```python
from build123d import *

# Parameters (mm, degrees)
F0_W     = 50
F0_H     = 50
F1_DEPTH = 400
F2_W     = 30
F2_H     = 30
F3_DEPTH = 40
F4_W     = 30
F4_H     = 10
F5_DEPTH = 30


with BuildPart() as f1:
    # F0 (on Top) → F1 (new body)
    with BuildSketch(Plane.XY):
        with Locations((-25, -25)):
            Rectangle(F0_W, F0_H)
    extrude(amount=-F1_DEPTH)

    # F2 (on face) → F3 (join)
    with BuildSketch(Plane.XY):
        with Locations((-25, -25)):
            Rectangle(F2_W, F2_H)
    extrude(amount=F3_DEPTH)

    # F4 (on face) → F5 (cut)
    with BuildSketch(Plane.XY.offset(40)):
        with Locations((-25, -35)):
            Rectangle(F4_W, F4_H)
        with Locations((-25, -15)):
            Rectangle(F4_W, F4_H)
    extrude(amount=-F5_DEPTH, mode=Mode.SUBTRACT)


solid = f1.part
```
Design review of the part built by this model. Coordinates are the model's own, in mm. A direction names the side the tool comes from. Round coordinates to 2 decimals unless told otherwise and drop trailing zeros. Order: outer loops, then holes, each group sorted by start corner. A loop starts at its lowest first (then second) coordinate and runs counter-clockwise, first axis right, second up. Notation, with made-up numbers: (-12.5, 2.25) - (41.5, 2.25) arc R15 ccw to (41.5, 31.25) - close; hole circle Ø6 at (2, 82.25). An arc over 180 degrees is marked (long way). One line per question, with ' | ' between items.
Item 1: Wall thickness on line 1 (Z direction, x = -18, y = -16); line 2 (Z direction, x = -8, y = -46.5); line 3 (X direction, y = -23, z = 5): over which ranges is each line inside the solid? List them lowest first. Write a range as [from, to].
Checks:
line 1: [-400, 10] | line 2: [-400, 0] | line 3: [-40, -10]
Item 2: Machinability: for faces 1 (the face through (-25, 0, -197)), 2 (the face through (-25, -40, 5)), 3 (the face through (-25, -10, 5)), which of the approach directions +Z, -Z, +X, -X, +Y, -Y give a long, thin tool a straight path to every point of the face, cutting with its end or side? Answer none if there is none.
Checks:
face 1: +Z, -Z, +X, -X, +Y | face 2: +Z, +X, -X, -Y | face 3: +Z, +X, -X, +Y
Item 3: For P1, Ø5, axis at x = -28, y = -36, coming from the +Z side; P2, Ø8, axis at x = -24, z = 6, coming from the +Y side; P3, Ø8, axis at x = -23.5, z = 5, coming from the -Y side, all flat-tipped, find the tip position at first contact; note any pin that passes through.
Checks:
P1: z = 10 | P2: y = -10 | P3: y = -40
Item 4: Take a section at B-B, the plane x = -45. Write out the cut boundary in (y, z).
Checks:
outline: (-50, -400) - (0, -400) - (0, 0) - (-50, 0) - close
Item 5: Draft analysis for pull direction X (two halves, no side actions). For faces 4 (the face through (-25, -41, 0)), 5 (the face through (-40, -25, 15)), 6 (the face through (-10, -25, 15)), state which applies: +X half, -X half, draft (parallel to the pull), parting line (faces both ways), or undercut.
Checks:
face 4: draft | face 5: -X half | face 6: +X half
Item 6: Take a section at A-A, the plane x = -29. Write out the cut boundary in (y, z), then the cut area to 3 significant figures.
Checks:
outline: (-50, -400) - (0, -400) - (0, 0) - (-10, 0) - (-10, 10) - (-20, 10) - (-20, 40) - (-30, 40) - (-30, 10) - (-40, 10) - (-40, 0) - (-50, 0) - close | area: 20,600 mm²
